Autodesk Inventor part; units mm, degrees
ref_plane "YZ Plane" through (0, 0, 0) normal (1, 0, 0) x (0, 1, 0)
ref_plane "XZ Plane" through (0, 0, 0) normal (0, 1, 0) x (-1, 0, 0)
ref_plane "XY Plane" through (0, 0, 0) normal (0, 0, 1) x (1, 0, 0)
sketch "Sketch1" plane through (0, 0, 0) normal (0, 1, 0) x (-1, 0, 0)
  line L0 (-20.05, 8.875) -> (20.05, 8.875)
  line L1 (20.05, 8.875) -> (20.05, -8.875)
  line L2 (20.05, -8.875) -> (-20.05, -8.875)
  line L3 (-20.05, -8.875) -> (-20.05, 8.875)
  line L4 (-20.05, 8.875) -> (20.05, -8.875) construction
  line L5 (20.05, 8.875) -> (-20.05, -8.875) construction
  point P0 (0, 0)
  dimension "d0" = 40
  dimension "d1" = 18
extrude "Extrusion1" add sketch "Sketch1" along normal blind 1.6
sketch "Sketch2" plane through (0, 1.6, 0) normal (0, 1, 0) x (1, 0, 0)
  line L0 (-2.5, -4.25) -> (2.5, -4.25)
  line L1 (2.5, -4.25) -> (2.5, 4.25)
  line L2 (2.5, 4.25) -> (-2.5, 4.25)
  line L3 (-2.5, 4.25) -> (-2.5, -4.25)
  line L4 (-2.5, -4.25) -> (2.5, 4.25) construction
  line L5 (2.5, -4.25) -> (-2.5, 4.25) construction
  point P0 (0, 0)
  dimension "d7" = 5
  dimension "d8" = 8.5
sketch "Sketch3" plane through (0, 1.6, 0) normal (0, 1, 0) x (1, 0, 0)
  circle A0 centre (-18.8, 7.625) radius 0.5
  line L0 (20.05, 8.875) -> (-20.05, 8.875)
  line L1 (-20.05, 8.875) -> (-20.05, -8.875)
  circle A1 centre (-16.3, 7.625) radius 0.5
  circle A2 centre (-13.8, 7.625) radius 0.5
  circle A3 centre (-11.3, 7.625) radius 0.5
  circle A4 centre (-8.8, 7.625) radius 0.5
  circle A5 centre (-6.3, 7.625) radius 0.5
  circle A6 centre (-3.8, 7.625) radius 0.5
  circle A7 centre (-1.3, 7.625) radius 0.5
  circle A8 centre (1.2, 7.625) radius 0.5
  circle A9 centre (3.7, 7.625) radius 0.5
  circle A10 centre (6.2, 7.625) radius 0.5
  circle A11 centre (8.7, 7.625) radius 0.5
  circle A12 centre (11.2, 7.625) radius 0.5
  circle A13 centre (13.7, 7.625) radius 0.5
  circle A14 centre (16.2, 7.625) radius 0.5
  circle A15 centre (18.7, 7.625) radius 0.5
  line L2 (-20.05, 0) -> (20.05, 0) construction
  line L3 (20.05, -8.875) -> (20.05, 8.875) construction
  circle A16 centre (-8.8, -7.625) radius 0.5
  circle A17 centre (-6.3, -7.625) radius 0.5
  circle A18 centre (-3.8, -7.625) radius 0.5
  circle A19 centre (-1.3, -7.625) radius 0.5
  circle A20 centre (1.2, -7.625) radius 0.5
  circle A21 centre (3.7, -7.625) radius 0.5
  circle A22 centre (6.2, -7.625) radius 0.5
  circle A23 centre (8.7, -7.625) radius 0.5
  circle A24 centre (-17.55, -6.375) radius 1.75
  line L4 (-20.05, -8.875) -> (20.05, -8.875)
  line L5 (0, 8.875) -> (0, -8.875) construction
  circle A25 centre (17.55, -6.375) radius 1.75
  point P0 (0, 0)
  dimension "d9" = 1
  dimension "d10" = 1.25
  dimension "d11" = 1.25
  dimension "d14" = 2.5
  dimension "d21" = 3.5
  dimension "d22" = 2.5
  dimension "d23" = 2.5
extrude "Extrusion2" cut sketch "Sketch3" against normal through all
properties part number "HW-178"
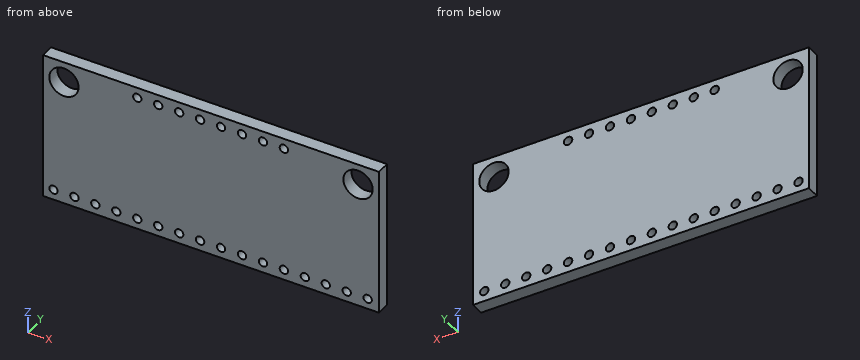
Input: part model. Units: mm. Frame: model coordinates. Coordinates: 2 decimals unless noted, no trailing zeros. Write each loop counter-clockwise with the first axis right and the second up, starting at its lowest first coordinate (ties: lowest second). Pieces come first, ordered by that corner, then holes.
1) Section A-A on x = 13.7. Output: boundary loops of the cut face in (y, z) (3 decimals).
2) Section C-C on y = 0.75. State how many separate pieces and enclosed holes the cut face has, and give its area (3 significant figures).
3) Material intervals for line 1 along Z through (x, y) = (-6.3, 0.4) (3 decimals); line 2 along X through (y, z) = (0.6, 5.5); line 3 along Z through (x, y) = (18.7, 0.7) (3 decimals), sorted ascending.
4) Section B-B on x = -3.8. Output: boundary loops of the cut face in (y, z) (3 decimals).
Check result:
1. outline: (0, -8.875) - (1.6, -8.875) - (1.6, -8.125) - (0, -8.125) - close; (0, -7.125) - (1.6, -7.125) - (1.6, 8.875) - (0, 8.875) - close
2. separate pieces: 1
2. enclosed holes: 26
2. area: 674 mm2
3. line 1: z = -8.875 to -8.125, -7.125 to 7.125, 8.125 to 8.875
3. line 2: x = -20.05 to -19.07, -16.03 to 16.03, 19.07 to 20.05
3. line 3: z = -8.875 to -8.125, -7.125 to 5.056, 7.694 to 8.875
4. outline: (0, -8.875) - (1.6, -8.875) - (1.6, -8.125) - (0, -8.125) - close; (0, -7.125) - (1.6, -7.125) - (1.6, 7.125) - (0, 7.125) - close; (0, 8.125) - (1.6, 8.125) - (1.6, 8.875) - (0, 8.875) - close
